Source: CAD feature listing. Evaluate the final solid. Frame: model axes, mm. A direction names the side the tool comes from. Round coordinates to 2 decimals unless told otherwise and drop trailing zeros. Loops run counter-clockwise (first coordinate to the right, second up) from the corner with the lowest first, then second, coordinate; pieces in that order, holes last. Notation, with made-up numbers: (24, 69.5) -> (48, 69.5) arc R25 ccw to (48, 85.5) -> close; hole circle Ø10 at (-10.5, 3). An arc over 180 degrees is marked (long way). Write item = value, one per line.
from build123d import *

# Parameters (mm, degrees)
SKETCH1_R               = 1
BOSS_EXTRUDE1_DEPTH     = 1.6
BOSS_EXTRUDE1_2_DEPTH   = 1.6
BOSS_EXTRUDE1_3_DEPTH   = 1.6
BOSS_EXTRUDE1_4_DEPTH   = 1.6
SKETCH2_R               = 1.5
BOSS_EXTRUDE2_DEPTH     = 1.5
BOSS_EXTRUDE3_DEPTH     = 2
SKETCH4_W               = 22.65
SKETCH4_H               = 30.55
BOSS_EXTRUDE4_DEPTH     = 6.6
SKETCH5_W               = 8.5
SKETCH5_H               = 3
CUT_EXTRUDE1_DEPTH      = 3.75
FILLET1_R               = 1
SKETCH6_R               = 5
CUT_EXTRUDE2_DEPTH      = 9
SKETCH8_R               = 5
CUT_EXTRUDE3_DEPTH      = 0.5
CUT_EXTRUDE3_DEPTH_BACK = 9
SKETCH9_W               = 22.65
SKETCH9_H               = 30.55
CUT_EXTRUDE4_DEPTH      = 1.6


with BuildPart() as part:
    # Sketch1 → Boss-Extrude1 (new body)
    with BuildSketch(Plane(origin=(0, 0.8, 0), x_dir=(1, 0, 0), z_dir=(0, 1, 0))):
        with Locations((-8.9, -13.05)):
            Circle(SKETCH1_R)
    extrude(amount=-BOSS_EXTRUDE1_DEPTH)



with BuildPart() as body_2:
    # Sketch1 → Boss-Extrude1 2 (new body)
    with BuildSketch(Plane(origin=(0, 0.8, 0), x_dir=(1, 0, 0), z_dir=(0, 1, 0))):
        with Locations((-8.9, 8.55)):
            Circle(SKETCH1_R)
    extrude(amount=-BOSS_EXTRUDE1_2_DEPTH)


with BuildPart() as body_3:
    # Sketch1 → Boss-Extrude1 3 (new body)
    with BuildSketch(Plane(origin=(0, 0.8, 0), x_dir=(1, 0, 0), z_dir=(0, 1, 0))):
        with Locations((8.9, 8.55)):
            Circle(SKETCH1_R)
    extrude(amount=-BOSS_EXTRUDE1_3_DEPTH)


with BuildPart() as body_4:
    # Sketch1 → Boss-Extrude1 4 (new body)
    with BuildSketch(Plane(origin=(0, 0.8, 0), x_dir=(1, 0, 0), z_dir=(0, 1, 0))):
        with Locations((8.9, -13.05)):
            Circle(SKETCH1_R)
    extrude(amount=-BOSS_EXTRUDE1_4_DEPTH)


with BuildPart() as part_1:
    add(part.part)

    add(body_2.part)  # Boss-Extrude2 merges body 2

    add(body_3.part)  # Boss-Extrude2 merges body 3

    add(body_4.part)  # Boss-Extrude2 merges body 4
    # Sketch2 → Boss-Extrude2 (add)
    with BuildSketch(Plane.XZ.offset(0.8)):
        with Locations((-8.9, -8.55)):
            Circle(SKETCH2_R)
        with Locations((-8.9, 13.05)):
            Circle(SKETCH2_R)
        with Locations((8.9, 13.05)):
            Circle(SKETCH2_R)
        with Locations((8.9, -8.55)):
            Circle(SKETCH2_R)
    extrude(amount=BOSS_EXTRUDE2_DEPTH)

    # Sketch3 → Boss-Extrude3 (add)
    with BuildSketch(Plane.XZ.offset(2.3)):
        Polygon((-15.325, 18.275), (15.325, 18.275), (15.325, 4.25), (11.825, 4.25), (11.825, -4.25), (15.325, -4.25), (15.325, -18.275), (-15.325, -18.275), (-15.325, -4.25), (-11.825, -4.25), (-11.825, 4.25), (-15.325, 4.25), align=None)
    extrude(amount=BOSS_EXTRUDE3_DEPTH)

    # Sketch4 → Boss-Extrude4 (add)
    with BuildSketch(Plane(origin=(0, -2.3, 0), x_dir=(1, 0, 0), z_dir=(0, 1, 0))):
        Polygon((-13.3, -16.75), (-4.2, -16.75), (-4.2, -18.275), (4.2, -18.275), (4.2, -16.75), (13.3, -16.75), (13.3, -4.5), (13.3, 4.5), (13.3, 16.75), (-13.3, 16.75), (-13.3, 4.5), (-13.3, -4.5), align=None)
        Rectangle(SKETCH4_W, SKETCH4_H, mode=Mode.SUBTRACT)
    extrude(amount=BOSS_EXTRUDE4_DEPTH)

    # Sketch5 → Cut-Extrude1 (cut)
    with BuildSketch(Plane(origin=(0, 4.3, 0), x_dir=(1, 0, 0), z_dir=(0, 1, 0))):
        with Locations((0, -16.775)):
            Rectangle(SKETCH5_W, SKETCH5_H)
    extrude(amount=-CUT_EXTRUDE1_DEPTH, mode=Mode.SUBTRACT)

    # Fillet1
    fillet1_edges = [part_1.edges().sort_by_distance(p)[0] for p in [
        (15.325, -3.3, 18.275),
        (-15.325, -3.3, 18.275),
        (-15.325, -3.3, -18.275),
        (15.325, -4.3, -11.2625),
        (15.325, -4.3, 11.2625),
        (0, -4.3, 18.275),
        (-15.325, -4.3, 11.2625),
        (-15.325, -4.3, -11.2625),
        (0, -4.3, -18.275),
        (15.325, -3.3, -18.275),
    ]]
    fillet(fillet1_edges, radius=FILLET1_R)

    # Sketch6 → Cut-Extrude2 (cut, through all)
    with BuildSketch(Plane(origin=(-7.325, 0, 0), x_dir=(0, 0, -1), z_dir=(1, 0, 0))):
        with Locations((-9.275, 5.95)):
            Circle(SKETCH6_R)
    extrude(amount=-CUT_EXTRUDE2_DEPTH, mode=Mode.SUBTRACT)

    # Sketch8 → Cut-Extrude3 (cut, two sides)
    with BuildSketch(Plane.XY.offset(-10.275)) as cut_extrude3_sk:
        with Locations((10.825, 5.95)):
            Circle(SKETCH8_R)
    extrude(amount=CUT_EXTRUDE3_DEPTH, mode=Mode.SUBTRACT)
    extrude(cut_extrude3_sk.sketch, amount=-CUT_EXTRUDE3_DEPTH_BACK, mode=Mode.SUBTRACT)

    # Sketch9 → Cut-Extrude4 (cut)
    with BuildSketch(Plane(origin=(0, 0.8, 0), x_dir=(1, 0, 0), z_dir=(0, 1, 0))):
        Rectangle(SKETCH9_W, SKETCH9_H)
    extrude(amount=-CUT_EXTRUDE4_DEPTH, mode=Mode.SUBTRACT)


solid = part_1.part
1. Contact query for flat-ended pins moving along their axis: pin 1 Ø4 at (y, z) = (-1.5, -8) entering from +X (3 decimals); pin 2 Ø2 at (x, y) = (-8.5, 2.5) entering from +Z; pin 3 Ø1.5 at (x, y) = (8.5, 3) entering from -Z (3 decimals); pin 4 Ø3 at (x, z) = (7, 10) entering from +Y. Output: stop coordinate, or through.
Evaluation:
pin_1 = 15.325
pin_2 = 16.75
pin_3 = 15.275
pin_4 = -2.3
2. Section query C-C (y = 3.25). Return the cut outline in (x, z) (3 decimals), then the cut area to 3 significant figures.
Evaluation:
outline = (-13.3, -16.75) -> (6.617, -16.75) -> (6.617, -15.275) -> (-11.325, -15.275) -> (-11.325, 5.067) -> (-13.3, 5.067) -> close; (-13.3, 13.483) -> (-11.325, 13.483) -> (-11.325, 15.275) -> (-4.25, 15.275) -> (-4.25, 16.75) -> (-13.3, 16.75) -> close; (4.25, 15.275) -> (11.325, 15.275) -> (11.325, -9.775) -> (13.3, -9.775) -> (13.3, 16.75) -> (4.25, 16.75) -> close
area = 149 mm²
3. Section query D-D (z = 2). Return the cut outline in (x, y) (3 decimals).
Evaluation:
outline = (-13.3, -2.3) -> (-11.825, -2.3) -> (-11.825, -4.3) -> (11.825, -4.3) -> (11.825, -2.3) -> (13.3, -2.3) -> (13.3, 4.3) -> (11.325, 4.3) -> (11.325, -2.3) -> (-11.325, -2.3) -> (-11.325, 4.3) -> (-13.3, 4.3) -> close
4. Section query B-B (x = -1). Return the cut outline in (y, z) (3 decimals), then the cut area to 3 significant figures.
Evaluation:
outline = (-4.3, -17.275) arc R1 ccw to (-3.3, -18.275) -> (-2.3, -18.275) -> (-2.3, -16.75) -> (4.3, -16.75) -> (4.3, -15.275) -> (-2.3, -15.275) -> (-2.3, 15.275) -> (0.55, 15.275) -> (0.55, 18.275) -> (-3.3, 18.275) arc R1 ccw to (-4.3, 17.275) -> close
area = 91.0 mm²
5. Line query: probe 1 along Z at (x, y) = (14, -2.5) (3 decimals); probe 2 along Z at (x, y) = (11, 0) (3 decimals); probe 3 along Z at (x, y) = (8.5, -1.25) (3 decimals). Output: solid intervals per line, ascending. Write a range as from..to.
Evaluation:
probe_1 = -18.275..-4.25, 4.25..18.275
probe_2 = -16.75..-15.275, 15.275..16.75
probe_3 = -16.75..-15.275, -9.996..-7.104, 11.604..14.496, 15.275..16.75
6. Mould query, pull axis X, two halves, no side actions, for faces 5 (the face through (10.92, 0.95, -15.54)), 6 (the face through (9, -0.8, 13)), 7 (the face through (0, -3, -18.275)), 8 (the face through (-15.024, -4.015, -10.671)). Classes: released by +X, released by -X, zero draft, split by the parting line, or undercut.
Evaluation:
face_5 = undercut
face_6 = undercut
face_7 = zero draft
face_8 = released by -X
7. Set-up query: faces 1 (the face through (13, -2.3, 0)), 2 (the face through (0, 1, -16.75)), 3 (the face through (9, 1, 16.75)), 4 (the face through (-4.2, -1, 18)). Return all of +Z, -Z, +X, -X, +Y, -Y with unobstructed straight access to the full face (end or side cutting, diameter ignored); none if empty.
Evaluation:
face_1 = +X, -Y
face_2 = -Z, +X, -X, +Y
face_3 = +Z, +X, +Y
face_4 = +Z, -X, +Y
8. Section query A-A (z = -8.55). Return the cut outline in (x, y) (3 decimals), then the cut area to 3 significant figures.
Evaluation:
outline = (-15.325, -3.3) arc R1 ccw to (-14.325, -4.3) -> (14.325, -4.3) arc R1 ccw to (15.325, -3.3) -> (15.325, -2.3) -> (13.3, -2.3) -> (13.3, 4.3) -> (11.325, 4.3) -> (11.325, -2.3) -> (10.4, -2.3) -> (10.4, -0.8) -> (7.4, -0.8) -> (7.4, -2.3) -> (-7.4, -2.3) -> (-7.4, -0.8) -> (-10.4, -0.8) -> (-10.4, -2.3) -> (-11.325, -2.3) -> (-11.325, 4.3) -> (-13.3, 4.3) -> (-13.3, -2.3) -> (-15.325, -2.3) -> close
area = 95.9 mm²
